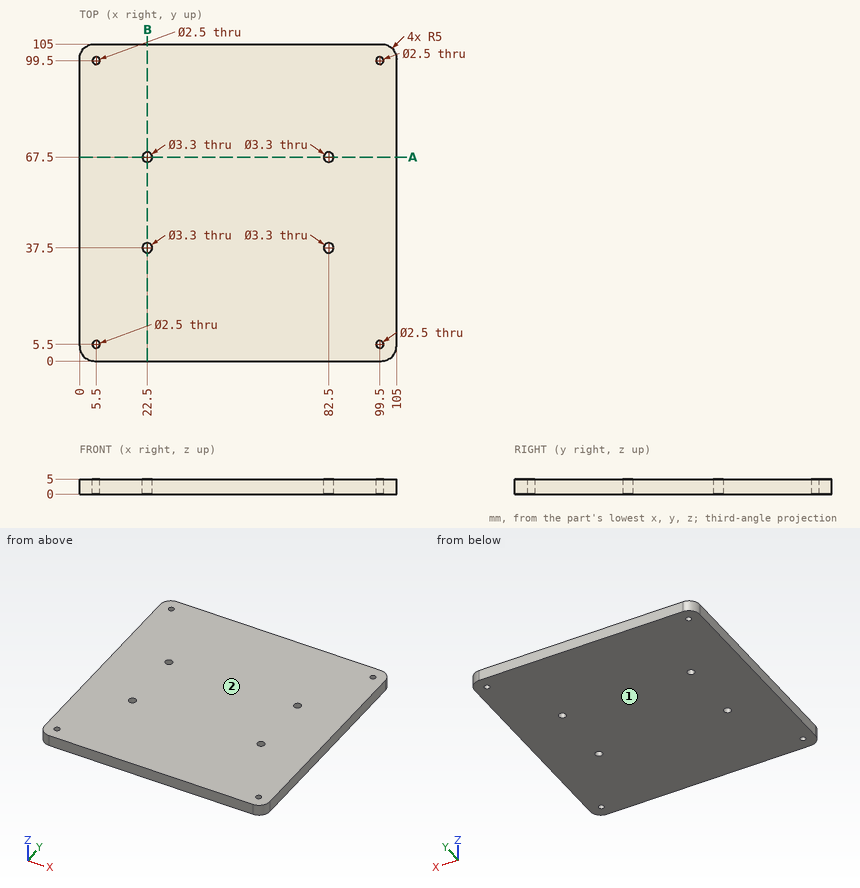
Geometry: see drawing. Coordinates: mm, zero at the bounding-box minimum. Round coordinates to 2 decimals unless told otherwise and drop trailing zeros. Write each loop counter-clockwise with the first axis right and the second up, starting at its lowest first coordinate (ties: lowest second). Pieces come first, ordered by that corner, then holes. Notation, with made-up numbers: (84, -34.75) -> (126, -34.75) arc R27 cw to (126, -15.75) -> close; hole circle Ø11 at (15.5, -33). An arc over 180 degrees is marked (long way). Answer as CSV lines item,"result".
1. Ray query, L1, parallel to Y at x = 99.5, z = 3.4; L2, parallel to Y at x = 22.5, z = 2.25. Return the intervals inside material, ascending. Write a range as [from, to].
Geometry says:
L1,"y = [0, 4.25], [6.75, 98.25], [100.75, 105]"
L2,"y = [0, 35.85], [39.15, 65.85], [69.15, 105]"
2. Section A-A (y = 67.5). Return the cut outline in (x, z).
Geometry says:
outline,"(0, 0) -> (20.85, 0) -> (20.85, 5) -> (0, 5) -> close; (24.15, 0) -> (80.85, 0) -> (80.85, 5) -> (24.15, 5) -> close; (84.15, 0) -> (105, 0) -> (105, 5) -> (84.15, 5) -> close"
3. Mould query, pull axis Z, two halves, no side actions, for the marked faces 1 and 2. Classes: +Z half, -Z half, draft (parallel to the pull), parting line (faces both ways), or undercut.
Geometry says:
face 1,"-Z half"
face 2,"+Z half"
4. Contact query for a flat-ended pin moving along its axis: P1, Ø3, axis at x = 82.5, y = 67.5, coming from the -Z side. Output: stop coordinate, or through.
Geometry says:
P1,"passes through"
5. Section B-B (x = 22.5). Return the cut outline in (y, z).
Geometry says:
outline,"(0, 0) -> (35.85, 0) -> (35.85, 5) -> (0, 5) -> close; (39.15, 0) -> (65.85, 0) -> (65.85, 5) -> (39.15, 5) -> close; (69.15, 0) -> (105, 0) -> (105, 5) -> (69.15, 5) -> close"
